Part model, mm, in its own coordinate system. Round coordinates to 2 decimals unless told otherwise and drop trailing zeros. Loops run counter-clockwise (first coordinate to the right, second up) from the corner with the lowest first, then second, coordinate; pieces in that order, holes last.
from build123d import *

# Parameters (mm, degrees)
F0_W           = 127
F0_H           = 101.6
F1_DEPTH       = 76.2
F3_D           = 12.7
F4_D           = 12.7
F4_DEPTH       = 12.7
F4_TIP         = 3.8154649308
F5_D           = 12.7
F5_CSINK_D     = 20.32
F5_CSINK_ANGLE = 82
F6_R           = 6.35
F7_DEPTH       = 25.4


with BuildPart() as f1:
    # F0 (on Top) → F1 (new body)
    with BuildSketch(Plane.XY):
        with Locations((8.4503423423, 0.4407010946)):
            Rectangle(F0_W, F0_H)
    extrude(amount=F1_DEPTH)

    # F3 (through all)
    with Locations(Plane.XY.offset(76.2)):
        with Locations((-32.9967327416, 33.7764918804)):
            Hole(F3_D / 2)

    # F4
    with Locations(Plane.XY.offset(76.2)):
        with Locations((7.6293125749, 33.5257202387)):
            Hole(F4_D / 2, depth=F4_DEPTH)
            with Locations((0, 0, -(F4_DEPTH + F4_TIP / 2))):  # 118° drill point
                Cone(0, F4_D / 2, F4_TIP, mode=Mode.SUBTRACT)

    # F5 (through all)
    with Locations(Plane.XY.offset(76.2)):
        with Locations((47.8257350624, 32.076139003)):
            CounterSinkHole(F5_D / 2, F5_CSINK_D / 2, counter_sink_angle=F5_CSINK_ANGLE)

    # F6 (on face) → F7 (cut)
    with BuildSketch(Plane.XY.offset(76.2)):
        with Locations((-29.4474586844, -21.6974113137)):
            Circle(F6_R)
    extrude(amount=-F7_DEPTH, mode=Mode.SUBTRACT)


solid = f1.part
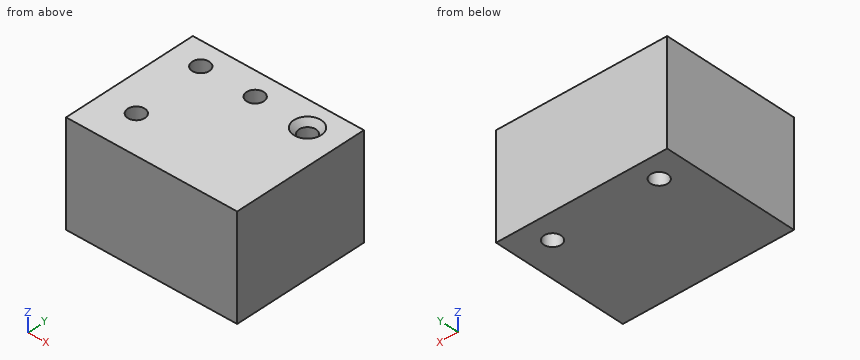
1) Slice it at B-B, the plane z = 14.5. Give the cut face in (x, y).
Values:
outline: (-55.05, -50.36) - (71.95, -50.36) - (71.95, 51.24) - (-55.05, 51.24) - close; hole circle Ø12.7 at (-33, 33.78); hole circle Ø12.7 at (47.83, 32.08)
2) Wall check: line 1 along X through (y, z) = (32, 6.5); line 2 along X through (y, z) = (31, 33); line 3 along Y through (x, z) = (-31, 72). Give the ranges that are in metal, low to high.
Values:
line 1: x = -55.05 to -39.09, -26.9 to 41.48, 54.18 to 71.95
line 2: x = -55.05 to -38.71, -27.29 to 41.57, 54.08 to 71.95
line 3: y = -50.36 to -27.85, -15.54 to 27.75, 39.8 to 51.24
3) Slice it at A-A, the plane z = 55.5. Give the cut face in (x, y).
Values:
outline: (-55.05, -50.36) - (71.95, -50.36) - (71.95, 51.24) - (-55.05, 51.24) - close; hole circle Ø12.7 at (-33, 33.78); hole circle Ø12.7 at (-29.45, -21.7); hole circle Ø12.7 at (47.83, 32.08)
4) Drop a flat-ended pin along its axis: pin 1 Ø7.5 at (x, y) = (-29.45, -21.7) entering from +Z. Give the stop position or say it passes through.
Values:
pin 1: stops at z = 50.8
